Part model, mm, in its own coordinate system. Face numbers are marked on the shaded views. Give positions to 0.01 mm unless a question says otherwise; leave off trailing zeros. Loops run counter-clockwise (first coordinate to the right, second up) from the corner with the lowest first, then second, coordinate; pieces in that order, holes last. Notation, with made-up numbers: (49.25, -9) -> (98.25, -9) arc R16 cw to (98.25, 13) -> close; hole circle Ø3 at (-5, 63.5). An arc over 180 degrees is marked (long way). One line per question, with ' | ' between items.
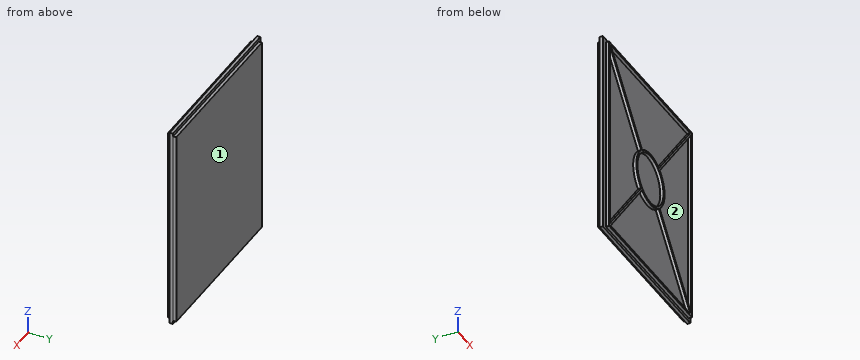
```python
from build123d import *

# Parameters (mm, degrees)
SKETCH1_W           = 203.2
SKETCH1_H           = 247.65
BOSS_EXTRUDE1_DEPTH = 3.81
SKETCH2_W           = 198.755
SKETCH2_H           = 240.03
BOSS_EXTRUDE2_DEPTH = 3.81
SKETCH3_W           = 192.405
SKETCH3_H           = 240.03
SKETCH3_W_2         = 188.332936508
SKETCH3_H_2         = 234.95
BOSS_EXTRUDE3_DEPTH = 3.81
SKETCH4_R           = 30.1625
BOSS_EXTRUDE4_DEPTH = 3.81


with BuildPart() as part:
    # Sketch1 → Boss-Extrude1 (new body)
    with BuildSketch(Plane(origin=(0, 0, 0), x_dir=(1, 0, 0), z_dir=(0, 1, 0))):
        with Locations((-1.5875, 0)):
            Rectangle(SKETCH1_W, SKETCH1_H)
    extrude(amount=BOSS_EXTRUDE1_DEPTH)

    # Sketch2 → Boss-Extrude2 (add)
    with BuildSketch(Plane(origin=(0, 3.81, 0), x_dir=(1, 0, 0), z_dir=(0, 1, 0))):
        Rectangle(SKETCH2_W, SKETCH2_H)
    extrude(amount=BOSS_EXTRUDE2_DEPTH)

    # Sketch3 → Boss-Extrude3 (add)
    with BuildSketch(Plane.XZ):
        Rectangle(SKETCH3_W, SKETCH3_H)
        Rectangle(SKETCH3_W_2, SKETCH3_H_2, mode=Mode.SUBTRACT)
    extrude(amount=BOSS_EXTRUDE3_DEPTH)

    # Sketch4 → Boss-Extrude4 (add)
    with BuildSketch(Plane(origin=(0, 0, 0), x_dir=(-1, 0, 0), z_dir=(0, -1, 0))):
        with BuildLine():
            Line((-92.538814631, 117.475), (-19.447411716, 26.291665671))
            ThreePointArc((-19.447411716, 26.291665671), (0, 32.7025), (19.447411716, 26.291665671))
            Line((19.447411716, 26.291665671), (92.538814631, 117.475))
            Line((92.538814631, 117.475), (94.166468254, 117.475))
            Line((94.166468254, 117.475), (94.166468254, 115.444461816))
            Line((94.166468254, 115.444461816), (21.429283015, 24.703022805))
            ThreePointArc((21.429283015, 24.703022805), (32.7025, 0), (21.429283015, -24.703022805))
            Line((21.429283015, -24.703022805), (94.166468254, -115.444461816))
            Line((94.166468254, -115.444461816), (94.166468254, -117.475))
            Line((94.166468254, -117.475), (92.538814631, -117.475))
            Line((92.538814631, -117.475), (19.447411716, -26.291665671))
            ThreePointArc((19.447411716, -26.291665671), (0, -32.7025), (-19.447411716, -26.291665671))
            Line((-19.447411716, -26.291665671), (-92.538814631, -117.475))
            Line((-92.538814631, -117.475), (-94.166468254, -117.475))
            Line((-94.166468254, -117.475), (-94.166468254, -115.444461816))
            Line((-94.166468254, -115.444461816), (-21.429283015, -24.703022805))
            ThreePointArc((-21.429283015, -24.703022805), (-32.7025, 0), (-21.429283015, 24.703022805))
            Line((-21.429283015, 24.703022805), (-94.166468254, 115.444461816))
            Line((-94.166468254, 115.444461816), (-94.166468254, 117.475))
            Line((-94.166468254, 117.475), (-92.538814631, 117.475))
        make_face()
        with Locations(Location((0, 0, 0), (0, 0, 90))):
            Circle(SKETCH4_R, mode=Mode.SUBTRACT)
    extrude(amount=BOSS_EXTRUDE4_DEPTH)


solid = part.part
```
1) Saw through at B-B (z = 0). Give the cut face in (x, y), and give its area (3 significant figures).
Found:
outline: (-103.19, 0) -> (-96.2, 0) -> (-96.2, -3.81) -> (-94.17, -3.81) -> (-94.17, 0) -> (-32.7, 0) -> (-32.7, -3.81) -> (-30.16, -3.81) -> (-30.16, 0) -> (30.16, 0) -> (30.16, -3.81) -> (32.7, -3.81) -> (32.7, 0) -> (94.17, 0) -> (94.17, -3.81) -> (96.2, -3.81) -> (96.2, 0) -> (100.01, 0) -> (100.01, 3.81) -> (99.38, 3.81) -> (99.38, 7.62) -> (-99.38, 7.62) -> (-99.38, 3.81) -> (-103.19, 3.81) -> close | area: 1,570 mm2
2) Pin check, flat tips, straight feed: P1, Ø1.1, axis at y = -1, z = -3, coming from the +X side; P2, Ø1.9, axis at y = -2.5, z = -53, coming from the -X side; P3, Ø4, axis at x = -8.5, y = -2.5, coming from the +Z side (3 decimals). Stop position of each tip, or through.
Found:
P1: x = 96.2 | P2: x = -96.2 | P3: z = 120.015
3) Saw through at A-A (x = 3.5). Give the cut face in (y, z) (3 decimals), and give its area (3 significant figures).
Found:
outline: (-3.81, -120.015) -> (0, -120.015) -> (0, -123.825) -> (3.81, -123.825) -> (3.81, -120.015) -> (7.62, -120.015) -> (7.62, 120.015) -> (3.81, 120.015) -> (3.81, 123.825) -> (0, 123.825) -> (0, 120.015) -> (-3.81, 120.015) -> (-3.81, 117.475) -> (0, 117.475) -> (0, 32.515) -> (-3.81, 32.515) -> (-3.81, 29.959) -> (0, 29.959) -> (0, -29.959) -> (-3.81, -29.959) -> (-3.81, -32.515) -> (0, -32.515) -> (0, -117.475) -> (-3.81, -117.475) -> close | area: 1,900 mm2
4) Pull direction X, two halves, no side cores. Call the marked faces 1 and 2: pulls with the +X half, pulls with the -X half, needs draft (parallel to the pull), parting line crosses it, or undercut.
Found:
face 1: needs draft | face 2: undercut
5) Drill centre lines: line 1 (Y direction, x = 45, z = -64); line 2 (X direction, y = -3, z = 27); line 3 (X direction, y = -1.75, z = -44.5). Where is each one in solid material? Low to high.
Found:
line 1: 0 to 7.62 | line 2: -96.2 to -94.17, -23.27 to -20.02, -18.45 to -13.45, 13.45 to 18.45, 20.02 to 23.27, 94.17 to 96.2 | line 3: -96.2 to -94.17, -37.3 to -34.04, 34.04 to 37.3, 94.17 to 96.2
